Verification items for the finished model (mm, model axes). Face numbers are marked on the shaded views. A direction names the side the tool comes from. Round coordinates to 2 decimals unless told otherwise and drop trailing zeros. Write each loop counter-clockwise with the first axis right and the second up, starting at its lowest first coordinate (ties: lowest second). Pieces come first, ordered by that corner, then holes. Notation, with made-up numbers: M 86,-6 L 136,-6 A21 ccw 136,0 Z; hole C 47.25,68 d8. An arc over 180 degrees is marked long. Write each question's results on one line, items separated by ' | '.
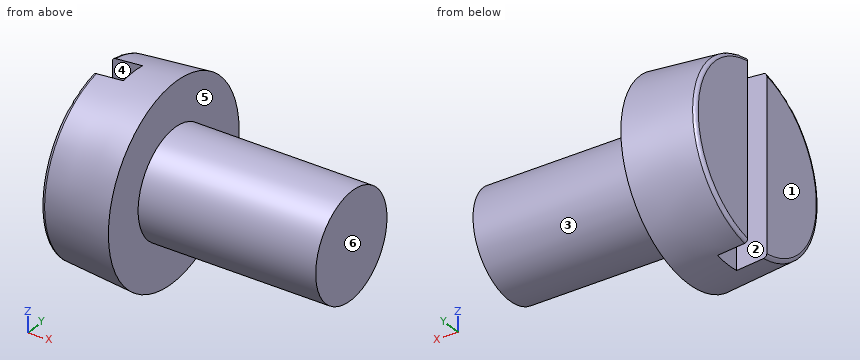
from build123d import *

# Parameters (mm, degrees)
FILLET2_R  = 0.1
SKETCH2_W  = 5.5
SKETCH2_H  = 0.8
SLOT_DEPTH = 0.85


with BuildPart() as part:
    # BodySke → Base-Revolve (revolve)
    with BuildSketch(Plane.XY):
        Polygon((2, 1.5), (2, 2.75), (0, 2.575022673), (0, 0), (7, 0), (7, 1.5), align=None)
    revolve(axis=Axis((-25.4, 0, 0), (1, 0, 0)))

    # Fillet2
    fillet2_edges = [part.edges().sort_by_distance(p)[0] for p in [
        (0, -2.575022673, 0),
    ]]
    fillet(fillet2_edges, radius=FILLET2_R)

    # Sketch2 → Slot (cut)
    with BuildSketch(Plane(origin=(0, 0, 0), x_dir=(0, 0, -1), z_dir=(1, 0, 0))):
        Rectangle(SKETCH2_W, SKETCH2_H)
    extrude(amount=SLOT_DEPTH, mode=Mode.SUBTRACT)


solid = part.part
1) Sectioned sample at D-D, the plane x = 4. Record the cut outline in (y, z).
Calculated:
outline: C 0,0 d3
2) Sectioned sample at A-A, the plane z = 0. Record the cut outline in (x, y).
Calculated:
outline: M 0,-2.48 A0.1 ccw 0.09,-2.58 L 2,-2.75 L 2,-1.5 L 7,-1.5 L 7,1.5 L 2,1.5 L 2,2.75 L 0.09,2.58 A0.1 ccw 0,2.48 L 0,0.4 L 0.85,0.4 L 0.85,-0.4 L 0,-0.4 Z
3) Access from +Z, -Z, +X, -X, +Y, -Y to the whole of each face (thin tool, end or side, straight path). Record for the marked faces 4, 5 and 6.
Calculated:
face 4: +Z, -Z, -X | face 5: +X | face 6: +Z, -Z, +X, +Y, -Y
4) Sectioned sample at B-B, the plane y = 0. Record the cut outline in (x, z), and give its area (3 significant figures).
Calculated:
outline: M 0.85,-2.65 L 2,-2.75 L 2,-1.5 L 7,-1.5 L 7,1.5 L 2,1.5 L 2,2.75 L 0.85,2.65 Z | area: 21.2 mm²
5) Material ranges on line 1 (X direction, y = -1.4, z = 1.9); line 2 (X direction, y = -0.1, z = 0.9); line 3 (Y direction, x = 3.75, z = -1.3), recorded low to high. Write a range as [from, to].
Calculated:
line 1: x = [0, 2] | line 2: x = [0.85, 7] | line 3: y = [-0.75, 0.75]
6) Depth check by flat-ended pin: P1, Ø0.6, axis at y = 0, z = -1, coming from the -X side; P2, Ø2, axis at x = 3.5, y = 0.5, coming from the -Z side. Enter the tip coordinate at first touch or a pass-through.
Calculated:
P1: stops at x = 0.85 | P2: stops at z = -1.5
7) Sectioned sample at C-C, the plane x = 0.5. Record the cut outline in (y, z), and give its area (3 significant figures).
Calculated:
outline: M -0.4,-2.59 L -0.4,2.59 A2.62 ccw Z; M 0.4,-2.59 A2.62 ccw 0.4,2.59 Z | area: 17.4 mm²
8) Draft check along Y on the marked faces 1, 2 and 3. Enter one of: pulls with the +Y half, pulls with the -Y half, needs draft (parallel to the pull), parting line crosses it, or undercut.
Calculated:
face 1: needs draft | face 2: undercut | face 3: parting line crosses it
